```python
from build123d import *

# Parameters (mm, degrees)
ESBO_O1_W      = 152
ESBO_O1_H      = 115
ESBO_O1_W_2    = 146.4
ESBO_O1_H_2    = 109.4
PAREDES_DEPTH  = 10
FILETE1_R      = 3
FILETE2_R      = 3
FILETE3_R      = 2
FILETE4_R      = 2
CHANFRO1_SIZE  = 3
CHANFRO2_SIZE  = 3
CHANFRO3_SIZE  = 5
CHANFRO4_SIZE  = 5
ESBO_O3_W      = 103.6
ESBO_O3_H      = 10
CORTES_DEPTH   = 10
FILETE7_RADIUS = 1.4
FILETE7_LENGTH = 10
FILETE8_RADIUS = 1.4
FILETE8_LENGTH = 10


with BuildPart() as part:
    # Esboço1 → Paredes (new body)
    with BuildSketch(Plane(origin=(0, 0, 0), x_dir=(1, 0, 0), z_dir=(0, 1, 0))):
        Rectangle(ESBO_O1_W, ESBO_O1_H)
        Rectangle(ESBO_O1_W_2, ESBO_O1_H_2, mode=Mode.SUBTRACT)
    extrude(amount=PAREDES_DEPTH)

    # Filete1
    filete1_edges = [part.edges().sort_by_distance(p)[0] for p in [
        (76, 5, 57.5),
    ]]
    fillet(filete1_edges, radius=FILETE1_R)

    # Filete2
    filete2_edges = [part.edges().sort_by_distance(p)[0] for p in [
        (-76, 5, 57.5),
    ]]
    fillet(filete2_edges, radius=FILETE2_R)

    # Filete3
    filete3_edges = [part.edges().sort_by_distance(p)[0] for p in [
        (76, 5, -57.5),
    ]]
    fillet(filete3_edges, radius=FILETE3_R)

    # Filete4
    filete4_edges = [part.edges().sort_by_distance(p)[0] for p in [
        (-76, 5, -57.5),
    ]]
    fillet(filete4_edges, radius=FILETE4_R)

    # Chanfro1
    chanfro1_edges = [part.edges().sort_by_distance(p)[0] for p in [
        (73.2, 5, 54.7),
    ]]
    chamfer(chanfro1_edges, length=CHANFRO1_SIZE)

    # Chanfro2
    chanfro2_edges = [part.edges().sort_by_distance(p)[0] for p in [
        (-73.2, 5, 54.7),
    ]]
    chamfer(chanfro2_edges, length=CHANFRO2_SIZE)

    # Chanfro3
    chanfro3_edges = [part.edges().sort_by_distance(p)[0] for p in [
        (-73.2, 5, -54.7),
    ]]
    chamfer(chanfro3_edges, length=CHANFRO3_SIZE)

    # Chanfro4
    chanfro4_edges = [part.edges().sort_by_distance(p)[0] for p in [
        (73.2, 5, -54.7),
    ]]
    chamfer(chanfro4_edges, length=CHANFRO4_SIZE)

    # Esboço3 → Cortes (cut)
    with BuildSketch(Plane(origin=(0, 0, -57.5), x_dir=(-1, 0, 0), z_dir=(0, 0, -1))):
        with BuildLine():
            Line((63.2, 6), (63.2, 4))
            ThreePointArc((63.2, 4), (62.760660172, 2.939339828), (61.7, 2.5))
            Line((61.7, 2.5), (59.7, 2.5))
            ThreePointArc((59.7, 2.5), (58.639339828, 2.939339828), (58.2, 4))
            Line((58.2, 4), (58.2, 6))
            ThreePointArc((58.2, 6), (58.639339828, 7.060660172), (59.7, 7.5))
            Line((59.7, 7.5), (61.7, 7.5))
            ThreePointArc((61.7, 7.5), (62.760660172, 7.060660172), (63.2, 6))
        make_face()
        with BuildLine():
            Line((-61.7, 7.5), (-59.7, 7.5))
            ThreePointArc((-59.7, 7.5), (-58.639339828, 7.060660172), (-58.2, 6))
            Line((-58.2, 6), (-58.2, 4))
            ThreePointArc((-58.2, 4), (-58.639339828, 2.939339828), (-59.7, 2.5))
            Line((-59.7, 2.5), (-61.7, 2.5))
            ThreePointArc((-61.7, 2.5), (-62.760660172, 2.939339828), (-63.2, 4))
            Line((-63.2, 4), (-63.2, 6))
            ThreePointArc((-63.2, 6), (-62.760660172, 7.060660172), (-61.7, 7.5))
        make_face()
        with Locations((0, 5)):
            Rectangle(ESBO_O3_W, ESBO_O3_H)
    extrude(amount=-CORTES_DEPTH, mode=Mode.SUBTRACT)

    # Filete7: full round fillet: the end face becomes a half cylinder, R = half its width
    filete7_face = Plane((51.8, 5, -56.1), x_dir=(0, 1, 0), z_dir=(-1, 0, 0))  # on the end face: x along it, z out of the body
    filete7_slab = filete7_face.offset(-FILETE7_RADIUS / 2) * Box(FILETE7_LENGTH, 2 * FILETE7_RADIUS, FILETE7_RADIUS, mode=Mode.PRIVATE)  # the body's end, R deep
    filete7_round = Plane((53.2, 5, -56.1), x_dir=(-1, 0, 0), z_dir=(0, 1, 0)) * Cylinder(FILETE7_RADIUS, FILETE7_LENGTH, mode=Mode.PRIVATE)  # its axis R under the face
    add(filete7_slab - filete7_round, mode=Mode.SUBTRACT)

    # Filete8: full round fillet: the end face becomes a half cylinder, R = half its width
    filete8_face = Plane((-51.8, 5, -56.1), x_dir=(0, -1, 0), z_dir=(1, 0, 0))  # on the end face: x along it, z out of the body
    filete8_slab = filete8_face.offset(-FILETE8_RADIUS / 2) * Box(FILETE8_LENGTH, 2 * FILETE8_RADIUS, FILETE8_RADIUS, mode=Mode.PRIVATE)  # the body's end, R deep
    filete8_round = Plane((-53.2, 5, -56.1), x_dir=(1, 0, 0), z_dir=(0, -1, 0)) * Cylinder(FILETE8_RADIUS, FILETE8_LENGTH, mode=Mode.PRIVATE)  # its axis R under the face
    add(filete8_slab - filete8_round, mode=Mode.SUBTRACT)


solid = part.part
```
Check sheet for the modelled part. Datum: model origin and axes. Units: mm. A direction names the side the tool comes from. Round coordinates to 2 decimals unless told otherwise and drop trailing zeros. Order: outer loops, then holes, each group sorted by start corner. A loop starts at its lowest first (then second) coordinate and runs counter-clockwise, first axis right, second up. Notation, with made-up numbers: (-8, 51.25) -> (23, 51.25) arc R16 ccw to (23, 61.25) -> close; hole circle Ø2 at (-32.5, 62.5). An arc over 180 degrees is marked (long way). One line per item, written item: value. Start each with the question number.
Q1. Cross-section at B-B (x = -3.5). Record the boundary of the cut face in (y, z).
Q2. Set-up check for faces 4 (the face through (-1, 5, 57.5)), 5 (the face through (-1, 5, 54.7)): record each of +Z, -Z, +X, -X, +Y, -Y from which the full face is reachable in a straight line by a thin tool's end or side.
Q3. Gauge pin test, flat ends, axial feed: pin 1 Ø3 at (x, y) = (-22, 3.5) entering from -Z; pin 2 Ø1 at (y, z) = (5, -56.5) entering from +X; pin 3 Ø1.6 at (y, z) = (4.5, -56.5) entering from -X. Record the tip position at first contact, or that the pin passes through.
Q4. Thickness scan on line 1 (X direction, y = 3.5, z = 13); line 2 (Z direction, x = 65, y = 5.25); line 3 (Z direction, x = 30.5, y = 5.25). Record the ranges inside material, lowest first.
Q5. Cross-section at A-A (z = 20.5). Record the boundary of the cut face in (x, y).
Q6. Mould release check, pull along X, two halves, no side actions. Record for faces 1 (the face through (63.5, 4.9, -57.5)), 2 (the face through (70.7, 4.9, -52.2)), 3 (the face through (76, 5, 0)): pulls with the +X half, pulls with the -X half, needs draft (parallel to the pull), parting line crosses it, or undercut.
Completed:
1. outline: (0, 54.7) -> (10, 54.7) -> (10, 57.5) -> (0, 57.5) -> close
2. face 4: +Z, +X, -X, +Y, -Y
2. face 5: +Y, -Y
3. pin 1: stops at z = 54.7
3. pin 2: stops at x = 75.94
3. pin 3: stops at x = -75.99
4. line 1: x = -76 to -73.2, 73.2 to 76
4. line 2: z = -57.5 to -54.7, 54.7 to 57.5
4. line 3: z = 54.7 to 57.5
5. outline: (-76, 0) -> (-73.2, 0) -> (-73.2, 10) -> (-76, 10) -> close; (73.2, 0) -> (76, 0) -> (76, 10) -> (73.2, 10) -> close
6. face 1: needs draft
6. face 2: undercut
6. face 3: pulls with the +X half
